from build123d import *

# Parameters (mm, degrees)
FILLET_1_R     = 1
CHAMFER_1_SIZE = 3


with BuildPart() as part:
    # 草图1 → 旋转1 (revolve)
    with BuildSketch(Plane.XY, mode=Mode.PRIVATE) as revolve_1_sk:
        Polygon((0, 0), (-120.5, 0), (-120.5, 17.5), (-163.5, 72.5), (-163.5, 87.5), (-148.5, 87.5), (-101, 40.5), (-101, 32.5), (0, 32.5), align=None)
    revolve(revolve_1_sk.sketch.rotate(Axis((-120.5, -37.5, 0), (1, 0, 0)), 90), axis=Axis((-120.5, -37.5, 0), (1, 0, 0)))

    # 圆角1
    fillet_1_edges = [part.edges().sort_by_distance(p)[0] for p in [
        (-101, -37.5, -70),
    ]]
    fillet(fillet_1_edges, radius=FILLET_1_R)

    # 倒角1
    chamfer_1_edges = [part.edges().sort_by_distance(p)[0] for p in [
        (0, -37.5, -70),
    ]]
    chamfer(chamfer_1_edges, length=CHAMFER_1_SIZE)


solid = part.part
Design review of the part built by this model. Coordinates are the model's own, in mm. A direction names the side the tool comes from. Give positions to 0.01 mm unless a question says otherwise; leave off trailing zeros. Write each loop counter-clockwise with the first axis right and the second up, starting at its lowest first coordinate (ties: lowest second). Pieces come first, ordered by that corner, then holes. Notation, with made-up numbers: M -17.75,50.25 L 28.25,50.25 A8 ccw 28.25,56.25 Z; hole C 1,21 d4. An arc over 180 degrees is marked long. Answer as a JSON object with one key per item and string values. Group by question number.
1) Mouldability with a two-part tool opening along Z and no side actions: class faces 4 (the face through (-61.09, -4.23, 17.3)), 5 (the face through (-0.15, -57.67, 64.05)), 6 (the face through (-163.5, 73, 1)) as released by +Z, released by -Z, zero draft, split by the parting line, or undercut.
2) Clearance check with flat-ended pins moving along their axes: pin 1 Ø6 at (x, z) = (-33.5, -51) entering from -Y; pin 2 Ø1.5 at (y, z) = (-46.5, -94.5) entering from -X; pin 3 Ø6 at (x, y) = (-21.5, -103.5) entering from -Z. State where each tip first meets the part, or that it passes through.
3) For line 1 along Y through (x, z) = (-33.5, 0); line 2 along Z through (x, y) = (-45, -37); line 3 along Y through (x, z) = (-154, -3.5), list the stretches that pass through material, from the lowest coordinate up.
4) We need section A-A (y = -37.5). Give the boundary of the cut face in (x, z), and give its area (3 significant figures).
5) Tool access review of faces 1 (the face through (-120.5, -26, -36)), 2 (the face through (-101, 31.5, -17.7)), 3 (the face through (-155.895, 38.561, -99.196)): name each direction out of +Z, -Z, +X, -X, +Y, -Y from which nothing blocks a thin tool from reaching the whole face with its end or side.
6) We need section B-B (z = 0). Give the boundary of the cut face in (x, y), and give its area (3 significant figures).
7) We need section D-D (x = -139). Give the boundary of the cut face in (y, z).
8) We need section C-C (x = -30.5). Give the boundary of the cut face in (y, z).
Answer key:
{
 "1": {"face 4": "undercut", "face 5": "split by the parting line", "face 6": "zero draft"},
 "2": {"pin 1": "stops at y = -88.45", "pin 2": "stops at x = -152.3", "pin 3": "stops at z = -30.51"},
 "3": {"line 1": "y = -107.5 to -75, 0 to 32.5", "line 2": "z = -70 to -37.5, 37.5 to 70", "line 3": "y = -162.45 to -135.29, 60.29 to 87.45"},
 "4": {"outline": "M -163.5,-125 L -148.5,-125 L -101,-78 L -101,-71 A1 cw -100,-70 L -3,-70 L 0,-67 L 0,-37.5 L -120.5,-37.5 L -120.5,-55 L -163.5,-110 Z; M -163.5,110 L -120.5,55 L -120.5,37.5 L 0,37.5 L 0,67 L -3,70 L -100,70 A1 cw -101,71 L -101,78 L -148.5,125 L -163.5,125 Z", "area": "11,400 mm²"},
 "5": {"face 1": "-X", "face 2": "+X", "face 3": "+X, -X"},
 "6": {"outline": "M -163.5,-162.5 L -148.5,-162.5 L -101,-115.5 L -101,-108.5 A1 cw -100,-107.5 L -3,-107.5 L 0,-104.5 L 0,-75 L -120.5,-75 L -120.5,-92.5 L -163.5,-147.5 Z; M -163.5,72.5 L -120.5,17.5 L -120.5,0 L 0,0 L 0,29.5 L -3,32.5 L -100,32.5 A1 cw -101,33.5 L -101,40.5 L -148.5,87.5 L -163.5,87.5 Z", "area": "11,400 mm²"},
 "7": {"outline": "C -37.5,0 d231.2; hole C -37.5,0 d157.33"},
 "8": {"outline": "C -37.5,0 d140; hole C -37.5,0 d75"}
}
